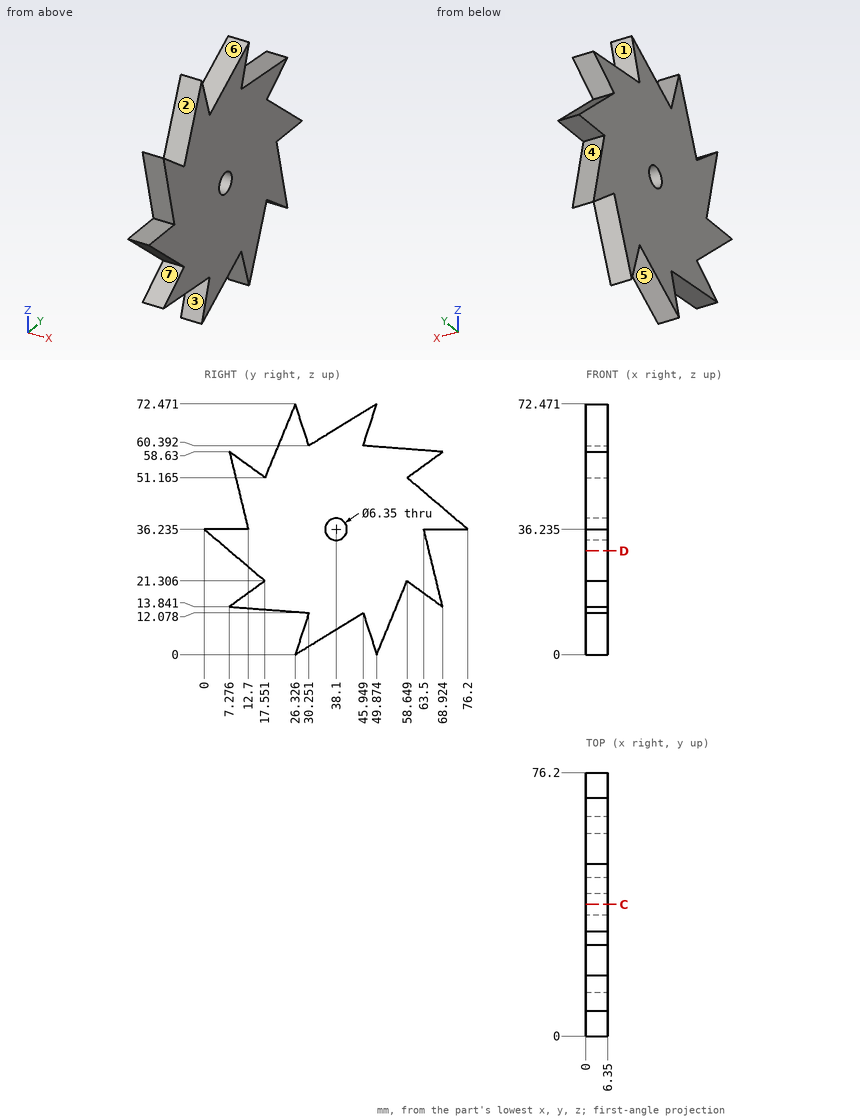
Design review of the part shown in the three views and the two pictorial views. Dimensions are in mm from the part's minimum x, y and z. A direction names the side the tool comes from. Give positions to 0.01 mm unless a question says otherwise; leave off trailing zeros. Order: outer loops, then holes, each group sorted by start corner. A loop starts at its lowest first (then second) coordinate and runs counter-clockwise, first axis right, second up. Notation, with made-up numbers: (38.25, 82.5) -> (75.25, 82.5) arc R34 cw to (75.25, 117.5) -> close; hole circle Ø5 at (77, -34.75). An arc over 180 degrees is marked (long way). Write each question's results on one line, items separated by ' | '. Start each with the question number.
Q1. Wall thickness on L1, parallel to Y at x = 1.5, z = 6 (1 decimal); L2, parallel to Z at x = 0.75, y = 60 (1 decimal); L3, parallel to Y at x = 5.5, z = 63.5 (1 decimal): over which ranges is each line inside the solid? List them lowest first. Write a range as from..to.
Q2. For pin 1 (1.5 mm diameter, centred on x = 1, y = 58, fed in from -Z) (1 decimal); pin 2 (3 mm diameter, centred on x = 5.5, y = 68, fed in from +Z); pin 3 (3 mm diameter, centred on x = 2.5, y = 7, fed in from +Z), all flat-tipped, find the tip position at first contact; note any pin that passes through.
Q3. Machinability: for the marked faces 4, 5, 6 and 7, which of the approach directions +Z, -Z, +X, -X, +Y, -Y give a long, thin tool a straight path to every point of the face, cutting with its end or side? Answer none if there is none.
Q4. Add section D-D on z = 30. Give the boundary of the cut face in (x, y).
Q5. Add section C-C on y = 38.1. Give the boundary of the cut face in (x, z), and give its area (3 significant figures).
Q6. Mouldability with a two-part tool opening along Y and no side actions: class the marked faces 1, 2 and 3 as +Y half, -Y half, draft (parallel to the pull), parting line (faces both ways), or undercut.
Found:
1) L1: y = 28.3..36.1, 47.9..52.3 | L2: z = 20.3..50, 52.1..59.3 | L3: y = 22.6..29.2, 35.3..47
2) pin 1: stops at z = 17.9 | pin 2: stops at z = 58.82 | pin 3: stops at z = 58.63
3) face 4: +X, -X, +Y | face 5: -Z, +X, -X | face 6: +Z, +X, -X | face 7: +X, -X, -Y
4) outline: (0, 7.33) -> (6.35, 7.33) -> (6.35, 65.01) -> (0, 65.01) -> close
5) outline: (0, 7.25) -> (6.35, 7.25) -> (6.35, 33.06) -> (0, 33.06) -> close; (0, 39.41) -> (6.35, 39.41) -> (6.35, 65.22) -> (0, 65.22) -> close | area: 328 mm2
6) face 1: +Y half | face 2: undercut | face 3: -Y half
